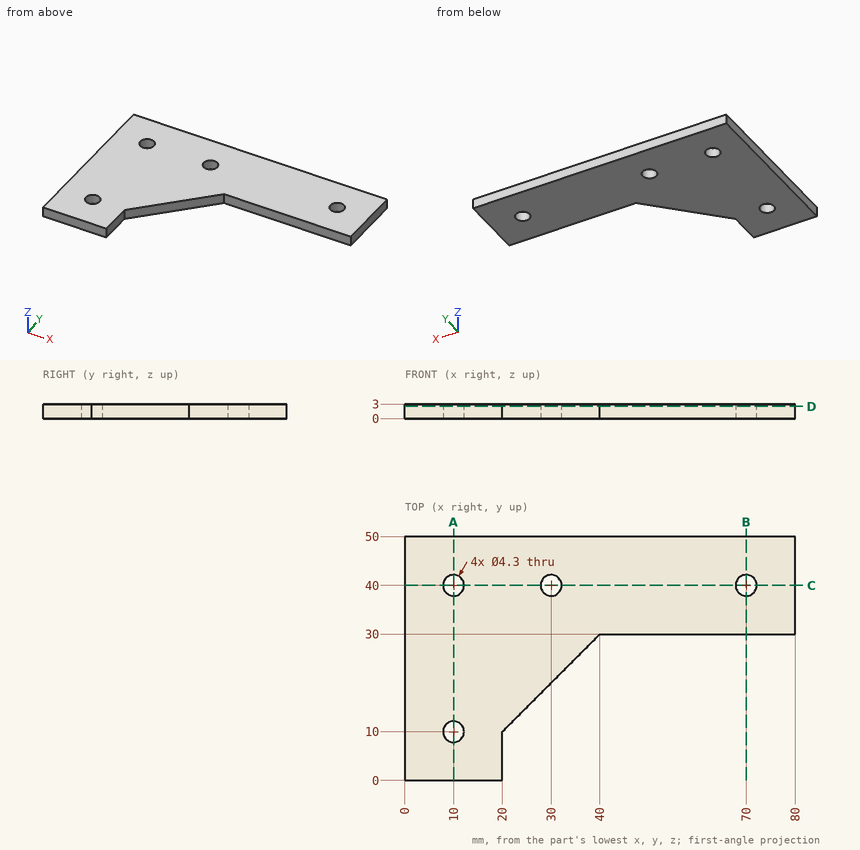
Could you check a few things on this drawing? It's one solid part, dimensions in mm from its lowest x, y, z. Round coordinates to 2 decimals unless told otherwise and drop trailing zeros. Loops run counter-clockwise (first coordinate to the right, second up) from the corner with the lowest first, then second, coordinate; pieces in that order, holes last. Notation, with made-up numbers: (-30.75, 68) -> (13.25, 68) arc R20 ccw to (13.25, 100) -> close; hole circle Ø9 at (77, -38.5). An arc over 180 degrees is marked (long way). Answer as CSV lines item,"result".
1. If we section it at D-D on z = 2.5: Please give me the cut outline in (x, y).
Final values:
outline,"(0, 0) -> (20, 0) -> (20, 10) -> (40, 30) -> (80, 30) -> (80, 50) -> (0, 50) -> close; hole circle Ø4.3 at (10, 10); hole circle Ø4.3 at (10, 40); hole circle Ø4.3 at (30, 40); hole circle Ø4.3 at (70, 40)"
2. If we section it at C-C on y = 40: Please give me the cut outline in (x, z), plus the area to 3 significant figures.
Final values:
outline,"(0, 0) -> (7.85, 0) -> (7.85, 3) -> (0, 3) -> close; (12.15, 0) -> (27.85, 0) -> (27.85, 3) -> (12.15, 3) -> close; (32.15, 0) -> (67.85, 0) -> (67.85, 3) -> (32.15, 3) -> close; (72.15, 0) -> (80, 0) -> (80, 3) -> (72.15, 3) -> close"
area,"201 mm^2"
3. If I drill on L1, parallel to Y at x = 10, z = 0.75; L2, parallel to Y at x = 30, z = 1.7; L3, parallel to Y at x = 8.5, z = 1.4, over which ranges is the centre line in solid material (lowest first)?
Final values:
L1,"y = 0 to 7.85, 12.15 to 37.85, 42.15 to 50"
L2,"y = 20 to 37.85, 42.15 to 50"
L3,"y = 0 to 8.46, 11.54 to 38.46, 41.54 to 50"
4. If we section it at B-B on x = 70: Please give me the cut outline in (y, z).
Final values:
outline,"(30, 0) -> (37.85, 0) -> (37.85, 3) -> (30, 3) -> close; (42.15, 0) -> (50, 0) -> (50, 3) -> (42.15, 3) -> close"
5. For pin 1 (4 mm diameter, centred on x = 10, y = 10, fed in from -Z), with a flat end and sliding along its axis, tell me the tip position at first contact or that it passes through.
Final values:
pin 1,"passes through"
6. If we section it at A-A on x = 10: Please give me the cut outline in (y, z).
Final values:
outline,"(0, 0) -> (7.85, 0) -> (7.85, 3) -> (0, 3) -> close; (12.15, 0) -> (37.85, 0) -> (37.85, 3) -> (12.15, 3) -> close; (42.15, 0) -> (50, 0) -> (50, 3) -> (42.15, 3) -> close"
